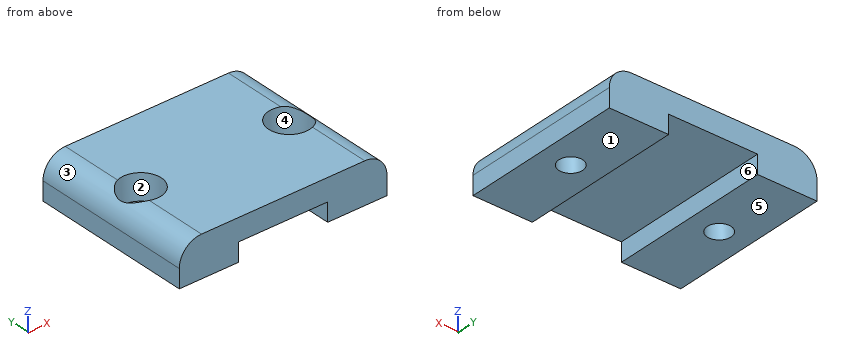
```python
from build123d import *

# Parameters (mm, degrees)
SKETCH1_W           = 28
SKETCH1_H           = 22
BOSS_EXTRUDE1_DEPTH = 3
SKETCH2_W           = 8
SKETCH2_H           = 22
BOSS_EXTRUDE2_DEPTH = 2.5
SKETCH3_R           = 1.6
CUT_EXTRUDE1_DEPTH  = 19.634645154
SKETCH4_R           = 2.75
CUT_EXTRUDE2_DEPTH  = 3.5
FILLET1_R           = 3


with BuildPart() as part:
    # Sketch1 → Boss-Extrude1 (new body)
    with BuildSketch(Plane.XY):
        Rectangle(SKETCH1_W, SKETCH1_H)
    extrude(amount=-BOSS_EXTRUDE1_DEPTH)

    # Sketch2 → Boss-Extrude2 (add)
    with BuildSketch(Plane(origin=(0, 0, -3), x_dir=(-1, 0, 0), z_dir=(0, 0, -1))):
        with Locations((10, 0)):
            Rectangle(SKETCH2_W, SKETCH2_H)
        with Locations((-10, 0)):
            Rectangle(SKETCH2_W, SKETCH2_H)
    extrude(amount=BOSS_EXTRUDE2_DEPTH)

    # Sketch3 → Cut-Extrude1 (cut, through all)
    with BuildSketch(Plane(origin=(0, 0, -5.5), x_dir=(-1, 0, 0), z_dir=(0, 0, -1))):
        with Locations((-10, 0)):
            Circle(SKETCH3_R)
        with Locations(Location((10, 0, 0), (0, 0, 180))):
            Circle(SKETCH3_R)
    extrude(amount=-CUT_EXTRUDE1_DEPTH, mode=Mode.SUBTRACT)

    # Sketch4 → Cut-Extrude2 (cut)
    with BuildSketch(Plane.XY):
        with Locations((-10, 0)):
            Circle(SKETCH4_R)
        with Locations((10, 0)):
            Circle(SKETCH4_R)
    extrude(amount=-CUT_EXTRUDE2_DEPTH, mode=Mode.SUBTRACT)

    # Fillet1
    # the kernel refuses this fillet: 3 mm, written as the material it takes off along each edge
    with BuildSketch(Plane(origin=(14, 18.5, 0), x_dir=(0, 0, -1), z_dir=(0, -1, 0)), Plane(origin=(-14, -18.5, 0), x_dir=(0, 0, -1), z_dir=(0, 1, 0))) as fillet1_piece_1:
        with BuildLine():
            CenterArc((FILLET1_R, -FILLET1_R), FILLET1_R, 90, 90)
            Line((0, -FILLET1_R), (0, 0))
            Line((0, 0), (FILLET1_R, 0))
        make_face()
    extrude(amount=37, mode=Mode.SUBTRACT)


solid = part.part
```
Design review of the part built by this model. Coordinates are the model's own, in mm. Face numbers are marked on the shaded views. A direction names the side the tool comes from. Give positions to 0.01 mm unless a question says otherwise; leave off trailing zeros. Write each loop counter-clockwise with the first axis right and the second up, starting at its lowest first coordinate (ties: lowest second). Pieces come first, ordered by that corner, then holes. Notation, with made-up numbers: (29.5, 16.25) - (88.5, 16.25) arc R8 ccw to (88.5, 30.25) - close; hole circle Ø7 at (8.25, 50). An arc over 180 degrees is marked (long way). Return JSON: item names as keys, results as strings. Group by question number.
(1) We need section C-C, the plane y = 7.5. Give the boundary of the cut face in (x, z), then the cut area to 3 significant figures.
(2) To check wall thickness, follow probe 1 along Y at (x, z) = (10, -4.25); probe 2 along X at (y, z) = (2.5, -5); probe 3 along Y at (x, z) = (-10, -2.8). State the ranges of each line that lie inside material, in increasing order.
(3) We need section A-A, the plane z = -4.5. Give the boundary of the cut face in (x, y), then the cut area to 3 significant figures.
(4) Insertion check: pin 1 (1.9 mm diameter, centred on x = 10, y = 0, fed in from +Z); pin 2 (1.6 mm diameter, centred on x = -10.5, y = -1.5, fed in from +Z). Each pin has a flat end and moves straight along its axis. Give the tip position at first contact, or say it passes through.
(5) Machinability: for the marked faces 4, 5 and 6, which of the approach directions +Z, -Z, +X, -X, +Y, -Y give a long, thin tool a straight path to every point of the face, cutting with its end or side? Answer none if there is none.
(6) We need section D-D, the plane z = -1.2. Give the boundary of the cut face in (x, y), then the cut area to 3 significant figures.
(7) We need section B-B, the plane x = -10. Give the boundary of the cut face in (y, z), then the cut area to 4 significant figures.
(8) Mouldability with a two-part tool opening along X and no side actions: class the marked faces 1, 2 and 3 as +X half, -X half, draft (parallel to the pull), parting line (faces both ways), or undercut.
Reported:
{
 "1": {"outline": "(-14, -5.5) - (-6, -5.5) - (-6, -3) - (6, -3) - (6, -5.5) - (14, -5.5) - (14, -3) arc R3 ccw to (11, 0) - (-11, 0) arc R3 ccw to (-14, -3) - close", "area": "120 mm2"},
 "2": {"probe 1": "y = -11 to -1.6, 1.6 to 11", "probe 2": "x = -14 to -6, 6 to 14", "probe 3": "y = -11 to -2.75, 2.75 to 11"},
 "3": {"outline": "(-14, -11) - (-6, -11) - (-6, 11) - (-14, 11) - close; (6, -11) - (14, -11) - (14, 11) - (6, 11) - close; hole circle Ø3.2 at (-10, 0); hole circle Ø3.2 at (10, 0)", "area": "336 mm2"},
 "4": {"pin 1": "passes through", "pin 2": "stops at z = -3.5"},
 "5": {"face 4": "+Z", "face 5": "-Z, +X, -X, +Y, -Y", "face 6": "-Z, +Y, -Y"},
 "6": {"outline": "(-13.4, -11) - (13.4, -11) - (13.4, 11) - (-13.4, 11) - close; hole circle Ø5.5 at (-10, 0); hole circle Ø5.5 at (10, 0)", "area": "542 mm2"},
 "7": {"outline": "(-11, -5.5) - (-1.6, -5.5) - (-1.6, -3.5) - (-2.75, -3.5) - (-2.75, 0) - (-11, 0) - close; (1.6, -5.5) - (11, -5.5) - (11, 0) - (2.75, 0) - (2.75, -3.5) - (1.6, -3.5) - close", "area": "95.35 mm2"},
 "8": {"face 1": "draft", "face 2": "undercut", "face 3": "-X half"}
}
